```python
from build123d import *

# Parameters (mm, degrees)
F0_R     = 11.2
F1_DEPTH = 9.7


with BuildPart() as f1:
    # F0 (on Top) → F1 (new body)
    with BuildSketch(Plane.XY):
        with BuildLine():
            ThreePointArc((10.7997121538, 2.9675271514), (11.9439907052, 1.4385768038), (13.2, 0))
            ThreePointArc((13.2, 0), (11.569588838, 6.3548889934), (7.0811190729, 11.1399170857))
            ThreePointArc((7.0811190729, 11.1399170857), (7.6213974776, 9.3082070065), (8.2978828887, 7.5223094569))
            ThreePointArc((8.2978828887, 7.5223094569), (9.8166208323, 5.3920270247), (10.7997121538, 2.9675271514))
        make_face()
        with BuildLine():
            ThreePointArc((12.6597128294, -3.7378698582), (13.0642299687, -1.8883578384), (13.2, 0))
            ThreePointArc((13.2, 0), (11.9439907052, 1.4385768038), (10.7997121538, 2.9675271514))
            ThreePointArc((10.7997121538, 2.9675271514), (11.0994769274, 1.4972013687), (11.2, 0))
            ThreePointArc((11.2, 0), (11.1797630339, -0.6729773444), (11.1191252668, -1.343522721))
            ThreePointArc((11.1191252668, -1.343522721), (11.861944996, -2.5583738361), (12.6597128294, -3.7378698582))
        make_face()
        with BuildLine():
            ThreePointArc((7.4945763109, 8.3229397403), (7.255524149, 9.7266841779), (7.0811190729, 11.1399170857))
            ThreePointArc((7.0811190729, 11.1399170857), (2.3229386222, 12.9939969277), (-2.7829079526, 12.9033105569))
            ThreePointArc((-2.7829079526, 12.9033105569), (-3.1202534931, 11.7668491168), (-3.4928140977, 10.641440207))
            ThreePointArc((-3.4928140977, 10.641440207), (2.312441633, 10.9586775522), (7.4945763109, 8.3229397403))
        make_face()
        with BuildLine():
            ThreePointArc((-2.7829079526, 12.9033105569), (2.3229386222, 12.9939969277), (7.0811190729, 11.1399170857))
            ThreePointArc((7.0811190729, 11.1399170857), (6.4857475715, 20.4865237167), (9.3208734987, 29.4126417821))
            ThreePointArc((9.3208734987, 29.4126417821), (-0.0838144074, 25.5596354988), (-9.4388150451, 29.5317602575))
            ThreePointArc((-9.4388150451, 29.5317602575), (-6.5025484684, 20.5664657708), (-7.0661295843, 11.1494310482))
            ThreePointArc((-7.0661295843, 11.1494310482), (-5.0019904472, 12.2155675908), (-2.7829079526, 12.9033105569))
        make_face()
        with BuildLine():
            ThreePointArc((8.2978828887, 7.5223094569), (7.6213974776, 9.3082070065), (7.0811190729, 11.1399170857))
            ThreePointArc((7.0811190729, 11.1399170857), (7.255524149, 9.7266841779), (7.4945763109, 8.3229397403))
            ThreePointArc((7.4945763109, 8.3229397403), (7.9063704761, 7.9327993732), (8.2978828887, 7.5223094569))
        make_face()
        with BuildLine():
            ThreePointArc((23.2557426949, -13.0949401652), (17.417829946, -9.0277901137), (12.6597128294, -3.7378698582))
            ThreePointArc((12.6597128294, -3.7378698582), (12.0939465538, -5.2892775267), (11.338902988, -6.7579049289))
            ThreePointArc((11.338902988, -6.7579049289), (8.4850698318, -10.1115572465), (4.6869245883, -12.3398840312))
            ThreePointArc((4.6869245883, -12.3398840312), (11.7287918196, -18.6207932863), (16.2380497133, -26.9095994984))
            ThreePointArc((16.2380497133, -26.9095994984), (17.5066070915, -18.8642279298), (23.2557426949, -13.0949401652))
        make_face()
        with BuildLine():
            ThreePointArc((11.338902988, -6.7579049289), (12.0939465538, -5.2892775267), (12.6597128294, -3.7378698582))
            ThreePointArc((12.6597128294, -3.7378698582), (11.861944996, -2.5583738361), (11.1191252668, -1.343522721))
            ThreePointArc((11.1191252668, -1.343522721), (10.3448630317, -4.2922964548), (8.8040757601, -6.9230231843))
            ThreePointArc((8.8040757601, -6.9230231843), (10.0695256921, -6.8103184234), (11.338902988, -6.7579049289))
        make_face()
        with BuildLine():
            ThreePointArc((-3.4928140977, 10.641440207), (-3.1202534931, 11.7668491168), (-2.7829079526, 12.9033105569))
            ThreePointArc((-2.7829079526, 12.9033105569), (-5.0019904472, 12.2155675908), (-7.0661295843, 11.1494310482))
            ThreePointArc((-7.0661295843, 11.1494310482), (-7.6009366797, 9.3278062246), (-8.271259726, 7.5515735145))
            ThreePointArc((-8.271259726, 7.5515735145), (-6.0815439879, 9.4050424094), (-3.4928140977, 10.641440207))
        make_face()
        with BuildLine():
            ThreePointArc((-9.4388150451, 29.5317602575), (-0.0838144074, 25.5596354988), (9.3208734987, 29.4126417821))
            ThreePointArc((9.3208734987, 29.4126417821), (12.1917088667, 33.6995042954), (13.2, 38.7593694031))
            ThreePointArc((13.2, 38.7593694031), (-4.9823509212, 50.9829604998), (-9.4388150451, 29.5317602575))
        make_face()
        with Locations((0, 38.7593694031)):
            Circle(F0_R, mode=Mode.SUBTRACT)
        with BuildLine():
            ThreePointArc((4.6869245883, -12.3398840312), (8.4850698318, -10.1115572465), (11.338902988, -6.7579049289))
            ThreePointArc((11.338902988, -6.7579049289), (10.0695256921, -6.8103184234), (8.8040757601, -6.9230231843))
            ThreePointArc((8.8040757601, -6.9230231843), (5.8741972555, -9.5359219063), (2.2226209928, -10.9772471924))
            ThreePointArc((2.2226209928, -10.9772471924), (3.4721946655, -11.6270584722), (4.6869245883, -12.3398840312))
        make_face()
        with BuildLine():
            ThreePointArc((42.4751993984, -24.8425416648), (36.1593540856, -13.5798415337), (23.2557426949, -13.0949401652))
            ThreePointArc((23.2557426949, -13.0949401652), (17.5066070915, -18.8642279298), (16.2380497133, -26.9095994984))
            ThreePointArc((16.2380497133, -26.9095994984), (16.6811751612, -28.3481754864), (17.0450643135, -29.8088074457))
            ThreePointArc((17.0450643135, -29.8088074457), (31.8052405917, -37.797806678), (42.4751993984, -24.8425416648))
        make_face()
        with Locations((29.2751993984, -24.8425416648)):
            Circle(F0_R, mode=Mode.SUBTRACT)
        with BuildLine():
            ThreePointArc((-8.271259726, 7.5515735145), (-7.6009366797, 9.3278062246), (-7.0661295843, 11.1494310482))
            ThreePointArc((-7.0661295843, 11.1494310482), (-11.5653125879, 6.3626680523), (-13.2, 0))
            ThreePointArc((-13.2, 0), (-11.947646657, 1.4268660523), (-10.8061773678, 2.9438971952))
            ThreePointArc((-10.8061773678, 2.9438971952), (-9.8129924989, 5.3986274383), (-8.271259726, 7.5515735145))
        make_face()
        with BuildLine():
            ThreePointArc((-4.589179085, -12.3765679946), (0.0522012849, -13.1998967809), (4.6869245883, -12.3398840312))
            ThreePointArc((4.6869245883, -12.3398840312), (3.4721946655, -11.6270584722), (2.2226209928, -10.9772471924))
            ThreePointArc((2.2226209928, -10.9772471924), (-0.1479208812, -11.1990231455), (-2.5117781872, -10.9147134794))
            ThreePointArc((-2.5117781872, -10.9147134794), (-3.5678638565, -11.6209350826), (-4.589179085, -12.3765679946))
        make_face()
        with BuildLine():
            ThreePointArc((17.0450643135, -29.8088074457), (16.6811751612, -28.3481754864), (16.2380497133, -26.9095994984))
            ThreePointArc((16.2380497133, -26.9095994984), (16.5586640372, -28.3822773057), (17.0450643135, -29.8088074457))
        make_face()
        with BuildLine():
            ThreePointArc((-10.8061773678, 2.9438971952), (-11.947646657, 1.4268660523), (-13.2, 0))
            ThreePointArc((-13.2, 0), (-13.0554049975, -1.9484353598), (-12.6247878255, -3.8541837476))
            ThreePointArc((-12.6247878255, -3.8541837476), (-11.7965458081, -3.0060317688), (-10.9951085748, -2.1325073104))
            ThreePointArc((-10.9951085748, -2.1325073104), (-11.192251242, 0.4165478802), (-10.8061773678, 2.9438971952))
        make_face()
        with BuildLine():
            ThreePointArc((-7.5366184006, -8.2848888396), (-9.7631539879, -5.4882441826), (-10.9951085748, -2.1325073104))
            ThreePointArc((-10.9951085748, -2.1325073104), (-11.7965458081, -3.0060317688), (-12.6247878255, -3.8541837476))
            ThreePointArc((-12.6247878255, -3.8541837476), (-11.6907811636, -6.1290811535), (-10.3510105514, -8.1912502442))
            ThreePointArc((-10.3510105514, -8.1912502442), (-8.9426172679, -8.2020863754), (-7.5366184006, -8.2848888396))
        make_face()
        with BuildLine():
            ThreePointArc((-14.2702107489, -27.6635521839), (-10.7633961504, -19.1754458925), (-4.589179085, -12.3765679946))
            ThreePointArc((-4.589179085, -12.3765679946), (-7.7576760542, -10.6798156463), (-10.3510105514, -8.1912502442))
            ThreePointArc((-10.3510105514, -8.1912502442), (-11.6907811636, -6.1290811535), (-12.6247878255, -3.8541837476))
            ThreePointArc((-12.6247878255, -3.8541837476), (-19.0361183181, -8.9729874739), (-26.3951306605, -12.5995902391))
            ThreePointArc((-26.3951306605, -12.5995902391), (-17.6733855055, -16.7701576999), (-14.1331403732, -25.7662199438))
            ThreePointArc((-14.1331403732, -25.7662199438), (-14.1674525628, -26.7173584612), (-14.2702107489, -27.6635521839))
        make_face()
        with BuildLine():
            ThreePointArc((-10.3510105514, -8.1912502442), (-7.7576760542, -10.6798156463), (-4.589179085, -12.3765679946))
            ThreePointArc((-4.589179085, -12.3765679946), (-3.5678638565, -11.6209350826), (-2.5117781872, -10.9147134794))
            ThreePointArc((-2.5117781872, -10.9147134794), (-5.1934153411, -9.923126377), (-7.5366184006, -8.2848888396))
            ThreePointArc((-7.5366184006, -8.2848888396), (-8.9426172679, -8.2020863754), (-10.3510105514, -8.1912502442))
        make_face()
        with BuildLine():
            ThreePointArc((-34.3061189534, -14.5582955275), (-34.5587070595, -36.8129925975), (-14.2702107489, -27.6635521839))
            ThreePointArc((-14.2702107489, -27.6635521839), (-14.1674525628, -26.7173584612), (-14.1331403732, -25.7662199438))
            ThreePointArc((-14.1331403732, -25.7662199438), (-17.6733855055, -16.7701576999), (-26.3951306605, -12.5995902391))
            ThreePointArc((-26.3951306605, -12.5995902391), (-30.2980685136, -13.7912117857), (-34.3061189534, -14.5582955275))
        make_face()
        with Locations((-27.3331403732, -25.7662199438)):
            Circle(F0_R, mode=Mode.SUBTRACT)
        with BuildLine():
            ThreePointArc((-34.3061189534, -14.5582955275), (-30.2980685136, -13.7912117857), (-26.3951306605, -12.5995902391))
            ThreePointArc((-26.3951306605, -12.5995902391), (-30.5055753859, -12.9531150862), (-34.3061189534, -14.5582955275))
        make_face()
    extrude(amount=F1_DEPTH)


solid = f1.part
```
Part model, mm, in its own coordinate system. A direction names the side the tool comes from. Round coordinates to 2 decimals unless told otherwise and drop trailing zeros. Loops run counter-clockwise (first coordinate to the right, second up) from the corner with the lowest first, then second, coordinate; pieces in that order, holes last.
Item 1: Mould opens along X. For faces 3 (the face through (-10.83, -19.28, 4.78)), 4 (the face through (-6.52, 20.7, 4.78)), 5 (the face through (-5.4, -10.1, 0)) say: +X half, -X half, draft (parallel to the pull), parting line (faces both ways), or undercut.
Item 2: Drill centre lines: line 1 (Y direction, x = -9, z = 6.25); line 2 (Y direction, x = -27, z = 0.5); line 3 (Y direction, x = -3, z = 4.5). Where is each one in solid material? Low to high.
Item 3: Drop flat-ended pins along their axis: P1, Ø2, axis at x = 24.5, z = 1.5, coming from the +Y side; P2, Ø2, axis at y = -7.5, z = 3.5, coming from the +X side; P3, Ø2, axis at x = -6.5, z = 3, coming from the +Y side. Give the stop position or say it passes through.
Item 4: Cut at D-D, the plane z = 1.25. Give the cut face in (x, y) (1 decimal), then the cut area to 3 significant figures.
Item 5: 3-axis set-ups, long thin cutter, end or side, ignore diameter. For faces 1 (the face through (21.02, -17.273, 4.782)), 2 (the face through (11.65, -18.52, 4.78)): which of +Z, -Z, +X, -X, +Y, -Y reach the whole face in a straight line?
Item 6: Cut at C-C, the plane y = -5. Give the cut face in (x, z), then the cut area to 3 significant figures.
Item 7: Cut at B-B, the plane x = -18.5. Give the cut face in (y, z).
Item 8: Cut at A-A, the plane x = 0. Give the cut face in (y, z).
A:
1. face 3: undercut
1. face 4: -X half
1. face 5: draft
2. line 1: y = -16.71 to -6.67, 6.67 to 9.66, 28.7 to 32.09, 45.43 to 48.42
2. line 2: y = -38.96 to -36.96, -14.57 to -12.57
2. line 3: y = -12.85 to -10.79, 10.79 to 27.97, 49.55 to 51.61
3. P1: stops at y = -12.19
3. P2: stops at x = 16.84
3. P3: stops at y = 50.76
4. outline: (-26.4, -12.6) arc R13.2 ccw (long way) to (-14.3, -27.7) arc R26.7 cw to (-4.6, -12.4) arc R13.2 ccw to (4.7, -12.3) arc R27.5 cw to (16.2, -26.9) arc R13.2 ccw (long way) to (23.3, -13.1) arc R31 cw to (12.7, -3.7) arc R13.2 ccw to (7.1, 11.1) arc R25.4 cw to (9.3, 29.4) arc R13.2 ccw (long way) to (-9.4, 29.5) arc R25.2 cw to (-7.1, 11.1) arc R13.2 ccw to (-12.6, -3.9) arc R38.1 cw to start; hole circle Ø22.4 at (-27.3, -25.8); hole circle Ø22.4 at (0, 0); hole circle Ø22.4 at (0, 38.8); hole circle Ø22.4 at (29.3, -24.8)
4. area: 1,110 mm2
5. face 1: +Z, -Z
5. face 2: +Z, -Z, -Y
6. outline: (-13.83, 0) - (-10.02, 0) - (-10.02, 9.7) - (-13.83, 9.7) - close; (10.02, 0) - (13.61, 0) - (13.61, 9.7) - (10.02, 9.7) - close
6. area: 71.7 mm2
7. outline: (-35.58, 0) - (-32.65, 0) - (-32.65, 9.7) - (-35.58, 9.7) - close; (-18.88, 0) - (-8.63, 0) - (-8.63, 9.7) - (-18.88, 9.7) - close
8. outline: (-13.2, 0) - (-11.2, 0) - (-11.2, 9.7) - (-13.2, 9.7) - close; (11.2, 0) - (27.56, 0) - (27.56, 9.7) - (11.2, 9.7) - close; (49.96, 0) - (51.96, 0) - (51.96, 9.7) - (49.96, 9.7) - close
